from build123d import *

# Parameters (mm, degrees)
ESBO_O1_W                = 195
ESBO_O1_H                = 195
RESSALTO_EXTRUS_O1_DEPTH = 10
ESBO_O2_W                = 7
ESBO_O2_H                = 32
ESBO_O2_W_2              = 32
ESBO_O2_H_2              = 7
CORTE_EXTRUS_O1_DEPTH    = 11
ESBO_O3_W                = 6.3
ESBO_O3_H                = 195
CORTE_EXTRUS_O2_DEPTH    = 4
ESBO_O4_R                = 1.5
CORTE_EXTRUS_O3_DEPTH    = 11
ESBO_O5_R                = 1.5
CORTE_EXTRUS_O4_DEPTH    = 11
ESBO_O6_R                = 7
CORTE_EXTRUS_O5_DEPTH    = 11
ESBO_O7_R                = 7
CORTE_EXTRUS_O6_DEPTH    = 7


with BuildPart() as part:
    # Esboço1 → Ressalto-extrusão1 (new body)
    with BuildSketch(Plane(origin=(0, 0, 0), x_dir=(1, 0, 0), z_dir=(0, 1, 0))):
        Rectangle(ESBO_O1_W, ESBO_O1_H)
    extrude(amount=RESSALTO_EXTRUS_O1_DEPTH)

    # Esboço2 → Corte-extrusão1 (cut, through all)
    with BuildSketch(Plane(origin=(0, 10, 0), x_dir=(1, 0, 0), z_dir=(0, 1, 0))):
        with Locations((-87.5, 47.5)):
            Rectangle(ESBO_O2_W, ESBO_O2_H)
        with Locations((-87.5, -47.5)):
            Rectangle(ESBO_O2_W, ESBO_O2_H)
        with Locations((-27.5, -92.5)):
            Rectangle(ESBO_O2_W_2, ESBO_O2_H_2)
        with Locations((47.5, -92.5)):
            Rectangle(ESBO_O2_W_2, ESBO_O2_H_2)
        with Locations((47.5, 92.5)):
            Rectangle(ESBO_O2_W_2, ESBO_O2_H_2)
        with Locations((-27.5, 92.5)):
            Rectangle(ESBO_O2_W_2, ESBO_O2_H_2)
    extrude(amount=-CORTE_EXTRUS_O1_DEPTH, mode=Mode.SUBTRACT)

    # Esboço3 → Corte-extrusão2 (cut)
    with BuildSketch(Plane(origin=(0, 10, 0), x_dir=(1, 0, 0), z_dir=(0, 1, 0))):
        with Locations((89.35, 0)):
            Rectangle(ESBO_O3_W, ESBO_O3_H)
    extrude(amount=-CORTE_EXTRUS_O2_DEPTH, mode=Mode.SUBTRACT)

    # Esboço4 → Corte-extrusão3 (cut, through all)
    with BuildSketch(Plane.XZ):
        with Locations((-87.5, 92.5)):
            Circle(ESBO_O4_R)
        with Locations((-87.5, -92.5)):
            Circle(ESBO_O4_R)
    extrude(amount=-CORTE_EXTRUS_O3_DEPTH, mode=Mode.SUBTRACT)

    # Esboço5 → Corte-extrusão4 (cut, through all)
    with BuildSketch(Plane.XZ):
        with Locations((75, 92.5)):
            Circle(ESBO_O5_R)
        with Locations((75, -92.5)):
            Circle(ESBO_O5_R)
    extrude(amount=-CORTE_EXTRUS_O4_DEPTH, mode=Mode.SUBTRACT)

    # Esboço6 → Corte-extrusão5 (cut, through all)
    with BuildSketch(Plane.XZ):
        with Locations((10, 0)):
            Circle(ESBO_O6_R)
    extrude(amount=-CORTE_EXTRUS_O5_DEPTH, mode=Mode.SUBTRACT)

    # Esboço7 → Corte-extrusão6 (cut)
    with BuildSketch(Plane(origin=(0, 10, 0), x_dir=(1, 0, 0), z_dir=(0, 1, 0))):
        Polygon((14.35, 7.534421013), (18.7, 0), (14.35, -7.534421013), (5.65, -7.534421013), (1.3, 0), (5.65, 7.534421013), align=None)
        with Locations((10, 0)):
            Circle(ESBO_O7_R, mode=Mode.SUBTRACT)
        with Locations((10, 0)):
            Circle(ESBO_O7_R)
    extrude(amount=-CORTE_EXTRUS_O6_DEPTH, mode=Mode.SUBTRACT)


solid = part.part
Verification items for the finished model (mm, model axes). A direction names the side the tool comes from. Round coordinates to 2 decimals unless told otherwise and drop trailing zeros. Loops run counter-clockwise (first coordinate to the right, second up) from the corner with the lowest first, then second, coordinate; pieces in that order, holes last. Notation, with made-up numbers: (-8.5, 26) - (36.5, 26) arc R17 ccw to (36.5, 44) - close; hole circle Ø8 at (2.5, 60.25). An arc over 180 degrees is marked (long way). Use a Markdown table: item, result. Add a question column.
1. Section check A-A, the plane z = -44. Record the boundary of the cut face in (x, y).
2. Access from +Z, -Z, +X, -X, +Y, -Y to the whole of each face (thin tool, end or side, straight path). Record for faces 1 (the face through (-1, 5, 97.5)), 2 (the face through (10, 7, 7.534)), 3 (the face through (63.5, 5, -92)).
3. Release check for a two-part mould opening along X. For faces 4 (the face through (-97.5, 5, 1)), 5 (the face through (-11.5, 5, 93)), 6 (the face through (-7, 10, -1)) record: released by +X, released by -X, zero draft, split by the parting line, or undercut.
4. Section check C-C, the plane x = 10. Record the boundary of the cut face in (y, z), plus the area to 3 significant figures.
5. Thickness scan on probe 1 along Z at (x, y) = (-14.5, 9); probe 2 along X at (y, z) = (8.75, -54.5); probe 3 along X at (y, z) = (2.75, -92.5). Record the ranges inside material, lowest first. Write a range as [from, to].
6. Section check B-B, the plane x = -40. Record the boundary of the cut face in (y, z), plus the area to 3 significant figures.
7. Gauge pin test, flat ends, axial feed: pin 1 (16.5 mm diameter, centred on x = 11.5, z = -3, fed in from +Y); pin 2 (2.5 mm diameter, centred on x = 75, z = -92.5, fed in from +Y). Record the tip position at first contact, or that the pin passes through.
Checks:
| question | item | result |
|---|---|---|
| 1 | outline | (-97.5, 0) - (-91, 0) - (-91, 10) - (-97.5, 10) - close; (-84, 0) - (97.5, 0) - (97.5, 10) - (92.5, 10) - (92.5, 6) - (86.2, 6) - (86.2, 10) - (-84, 10) - close |
| 2 | face 1 | +Z, +X, -X, +Y, -Y |
| 2 | face 2 | +Y |
| 2 | face 3 | +Y, -Y |
| 3 | face 4 | released by -X |
| 3 | face 5 | undercut |
| 3 | face 6 | zero draft |
| 4 | outline | (0, -97.5) - (10, -97.5) - (10, -7.53) - (3, -7.53) - (3, -7) - (0, -7) - close; (0, 7) - (3, 7) - (3, 7.53) - (10, 7.53) - (10, 97.5) - (0, 97.5) - close |
| 4 | area | 1,800 mm^2 |
| 5 | probe 1 | z = [-97.5, -96], [-89, 89], [96, 97.5] |
| 5 | probe 2 | x = [-97.5, -91], [-84, 86.2], [92.5, 97.5] |
| 5 | probe 3 | x = [-97.5, -89], [-86, -43.5], [-11.5, 31.5], [63.5, 73.5], [76.5, 97.5] |
| 6 | outline | (0, -97.5) - (10, -97.5) - (10, -96) - (0, -96) - close; (0, -89) - (10, -89) - (10, 89) - (0, 89) - close; (0, 96) - (10, 96) - (10, 97.5) - (0, 97.5) - close |
| 6 | area | 1,810 mm^2 |
| 7 | pin 1 | stops at y = 10 |
| 7 | pin 2 | passes through |
